Build history of the part. All positions in model axes, mm. Coordinates: 2 decimals unless noted, no trailing zeros. Write each loop counter-clockwise with the first axis right and the second up, starting at its lowest first coordinate (ties: lowest second). Pieces come first, ordered by that corner, then holes. Notation, with made-up numbers: (64.5, -3.75) -> (70.5, -3.75) arc R12 cw to (70.5, 0.25) -> close; hole circle Ø8 at (11, -30). An arc over 180 degrees is marked (long way). Write each question's results on one line, items separated by ' | '. Start each with the question number.
Q1. Saw through at A-A on x = 0. Give the cut face in (y, z), and give its area (3 significant figures).
Q2. Saw through at C-C on y = 18. Give the cut face in (x, z), and give its area (3 significant figures).
Q3. Saw through at B-B on z = 3.4. Give the cut face in (x, y), and give its area (3 significant figures).
Q4. Saw through at D-D on y = -47. Give the cut face in (x, z), and give its area (3 significant figures).
Q5. Drill centre lines: line 1 (X direction, y = -21, z = 5.7); line 2 (X direction, y = 13.5, z = 5.75); line 3 (X direction, y = -59, z = 3.05). Where is each one in solid material? Low to high.
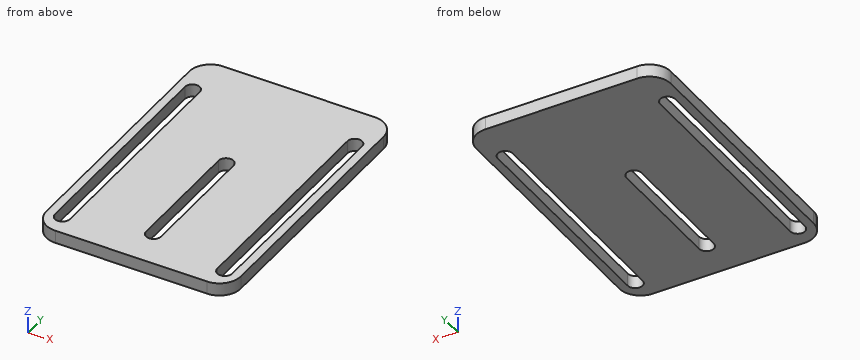
from build123d import *

# Parameters (mm, degrees)
BOSS_EXTRUDE1_DEPTH = 6


with BuildPart() as part:
    # Sketch1 → Boss-Extrude1 (new body)
    with BuildSketch(Plane.XY):
        with BuildLine():
            Line((-35.5, -67.136177844), (35.5, -67.136177844))
            ThreePointArc((35.5, -67.136177844), (42.571067812, -64.207245656), (45.5, -57.136177844))
            Line((45.5, -57.136177844), (45.5, 57.136177844))
            ThreePointArc((45.5, 57.136177844), (42.571067812, 64.207245656), (35.5, 67.136177844))
            Line((35.5, 67.136177844), (-35.5, 67.136177844))
            ThreePointArc((-35.5, 67.136177844), (-42.571067812, 64.207245656), (-45.5, 57.136177844))
            Line((-45.5, 57.136177844), (-45.5, -57.136177844))
            ThreePointArc((-45.5, -57.136177844), (-42.571067812, -64.207245656), (-35.5, -67.136177844))
        make_face()
        with BuildLine():
            Line((-34.5, 46.873645637), (-34.5, -57.136177844))
            ThreePointArc((-34.5, -57.136177844), (-38, -60.636177844), (-41.5, -57.136177844))
            Line((-41.5, -57.136177844), (-41.5, 46.873645637))
            ThreePointArc((-41.5, 46.873645637), (-38, 50.373645637), (-34.5, 46.873645637))
        make_face(mode=Mode.SUBTRACT)
        with BuildLine():
            Line((34.5, -57.136177844), (34.5, 46.873645637))
            ThreePointArc((34.5, 46.873645637), (38, 50.373645637), (41.5, 46.873645637))
            Line((41.5, 46.873645637), (41.5, -57.136177844))
            ThreePointArc((41.5, -57.136177844), (38, -60.636177844), (34.5, -57.136177844))
        make_face(mode=Mode.SUBTRACT)
        with BuildLine():
            Line((3.5, 8.791581559), (3.5, -49.136177844))
            ThreePointArc((3.5, -49.136177844), (0, -52.636177844), (-3.5, -49.136177844))
            Line((-3.5, -49.136177844), (-3.5, 8.791581559))
            ThreePointArc((-3.5, 8.791581559), (0, 12.291581559), (3.5, 8.791581559))
        make_face(mode=Mode.SUBTRACT)
    extrude(amount=BOSS_EXTRUDE1_DEPTH)


solid = part.part
Returned:
1) outline: (-67.14, 0) -> (-52.64, 0) -> (-52.64, 6) -> (-67.14, 6) -> close; (12.29, 0) -> (67.14, 0) -> (67.14, 6) -> (12.29, 6) -> close | area: 416 mm2
2) outline: (-45.5, 0) -> (-41.5, 0) -> (-41.5, 6) -> (-45.5, 6) -> close; (-34.5, 0) -> (34.5, 0) -> (34.5, 6) -> (-34.5, 6) -> close; (41.5, 0) -> (45.5, 0) -> (45.5, 6) -> (41.5, 6) -> close | area: 462 mm2
3) outline: (-45.5, -57.14) arc R10 ccw to (-35.5, -67.14) -> (35.5, -67.14) arc R10 ccw to (45.5, -57.14) -> (45.5, 57.14) arc R10 ccw to (35.5, 67.14) -> (-35.5, 67.14) arc R10 ccw to (-45.5, 57.14) -> close; hole (-41.5, -57.14) arc R3.5 ccw to (-34.5, -57.14) -> (-34.5, 46.87) arc R3.5 ccw to (-41.5, 46.87) -> close; hole (-3.5, -49.14) arc R3.5 ccw to (3.5, -49.14) -> (3.5, 8.79) arc R3.5 ccw to (-3.5, 8.79) -> close; hole (34.5, -57.14) arc R3.5 ccw to (41.5, -57.14) -> (41.5, 46.87) arc R3.5 ccw to (34.5, 46.87) -> close | area: 10,200 mm2
4) outline: (-45.5, 0) -> (-41.5, 0) -> (-41.5, 6) -> (-45.5, 6) -> close; (-34.5, 0) -> (-3.5, 0) -> (-3.5, 6) -> (-34.5, 6) -> close; (3.5, 0) -> (34.5, 0) -> (34.5, 6) -> (3.5, 6) -> close; (41.5, 0) -> (45.5, 0) -> (45.5, 6) -> (41.5, 6) -> close | area: 420 mm2
5) line 1: x = -45.5 to -41.5, -34.5 to -3.5, 3.5 to 34.5, 41.5 to 45.5 | line 2: x = -45.5 to -41.5, -34.5 to 34.5, 41.5 to 45.5 | line 3: x = -45.32 to -40.96, -35.04 to 35.04, 40.96 to 45.32
